```python
from build123d import *

# Parameters (mm, degrees)
SKETCH1_W                    = 140
SKETCH1_H                    = 1320
BASE_FLANGE1_DEPTH           = 10
EDGE_FLANGE1_STRIP_W         = 68
EDGE_FLANGE1_STRIP_H         = 10
EDGE_FLANGE1_STRIP_CUT_DEPTH = 1320
EDGE_FLANGE1_DEPTH           = 1320
SKETCH12_R                   = 10
CUT_EXTRUDE1_DEPTH           = 10
SKETCH13_R                   = 10
CUT_EXTRUDE2_DEPTH           = 10
LPATTERN1_COUNT              = 8
LPATTERN1_PITCH              = 152


# Sheet-metal steps are written as plain solids
with BuildPart() as part:
    # Sketch1 → Base-Flange1 (new body)
    with BuildSketch(Plane.XY):
        Rectangle(SKETCH1_W, SKETCH1_H)
    extrude(amount=-BASE_FLANGE1_DEPTH)

    # Edge-Flange1 strip (across the edge) → Edge-Flange1 strip cut (cut)
    with BuildSketch(Plane(origin=(70, -660, 0), x_dir=(-1, 0, 0), z_dir=(0, 1, 0))):
        with Locations((-10, -5)):
            Rectangle(EDGE_FLANGE1_STRIP_W, EDGE_FLANGE1_STRIP_H)
    extrude(amount=EDGE_FLANGE1_STRIP_CUT_DEPTH, mode=Mode.SUBTRACT)

    # Edge-Flange1 section (across the edge) → Edge-Flange1 (add)
    with BuildSketch(Plane(origin=(70, -660, 0), x_dir=(-1, 0, 0), z_dir=(0, 1, 0))):
        with BuildLine():
            Line((0, 14), (0, 140))
            Line((0, 140), (10, 140))
            Line((10, 140), (10, 14))
            ThreePointArc((10, 14), (14.100505063, 4.100505063), (24, 0))
            Line((24, 0), (24, -10))
            ThreePointArc((24, -10), (7.029437252, -2.970562748), (0, 14))
        make_face()
    extrude(amount=EDGE_FLANGE1_DEPTH)

    # Sketch12 → Cut-Extrude1 (cut)
    with BuildSketch(Plane.ZY.offset(-60)):
        with Locations((77, 532)):
            Circle(SKETCH12_R)
    cut_extrude1 = extrude(amount=-CUT_EXTRUDE1_DEPTH, mode=Mode.SUBTRACT)

    # Sketch13 → Cut-Extrude2 (cut)
    with BuildSketch(Plane.XY):
        with Locations((-7, 532)):
            Circle(SKETCH13_R)
    cut_extrude2 = extrude(amount=-CUT_EXTRUDE2_DEPTH, mode=Mode.SUBTRACT)

    # LPattern1: Cut-Extrude1, Cut-Extrude2 ×8
    with Locations(*[(0, -i * LPATTERN1_PITCH, 0) for i in range(1, LPATTERN1_COUNT)]):
        add(cut_extrude1, mode=Mode.SUBTRACT)
        add(cut_extrude2, mode=Mode.SUBTRACT)


solid = part.part
```
Check sheet for the modelled part. Datum: model origin and axes. Units: mm. A direction names the side the tool comes from. Round coordinates to 2 decimals unless told otherwise and drop trailing zeros. Order: outer loops, then holes, each group sorted by start corner. A loop starts at its lowest first (then second) coordinate and runs counter-clockwise, first axis right, second up. Notation, with made-up numbers: M -2,33.25 L 14,33.25 A28 cw 14,69.25 Z; hole C 22,-12 d2. An arc over 180 degrees is marked long. Answer in a Markdown table with one row per item.
(1) Set-up check for faces 1 (the flat face through (-13, 9, -10)), 2 (the flat face through (60, -9, 78)): record each of +Z, -Z, +X, -X, +Y, -Y from which the full face is reachable in a straight line by a thin tool's end or side.
Findings:
| item | result |
|---|---|
| face 1 | -Z, +X, -X, +Y, -Y |
| face 2 | +Z, -X, +Y, -Y |
(2) Material ranges on line 1 along X through (y, z) = (425, 119); line 2 along Z through (x, y) = (64, -380); line 3 along Z through (x, y) = (33.5, 15), recorded low to high. Write a range as from..to.
Findings:
| item | result |
|---|---|
| line 1 | x = 60..70 |
| line 2 | z = -1.87..67, 87..140 |
| line 3 | z = -10..0 |
(3) Gauge pin test, flat ends, axial feed: pin 1 (23 mm diameter, centred on y = 228, z = 77, fed in from -X); pin 2 (23 mm diameter, centred on x = -7, y = -380, fed in from +Z). Record the tip position at first contact, or that the pin passes through.
Findings:
| item | result |
|---|---|
| pin 1 | stops at x = 60 |
| pin 2 | stops at z = 0 |
(4) Section check A-A on y = 560. Record the boundary of the cut face in (x, z).
Findings:
| item | result |
|---|---|
| outline | M -70,-10 L 46,-10 A24 ccw 70,14 L 70,140 L 60,140 L 60,14 A14 cw 46,0 L -70,0 Z |
(5) Section check B-B on x = 14. Record the boundary of the cut face in (y, z).
Findings:
| item | result |
|---|---|
| outline | M -660,-10 L 660,-10 L 660,0 L -660,0 Z |
(6) Section check C-C on z = 119. Record the boundary of the cut face in (x, y), plus the area to 3 significant figures.
Findings:
| item | result |
|---|---|
| outline | M 60,-660 L 70,-660 L 70,660 L 60,660 Z |
| area | 13,200 mm^2 |
